Could you check a few things on this model? Use its own coordinates, in mm. Face numbers are marked on the shaded views. A direction names the side the tool comes from. Round coordinates to 2 decimals unless told otherwise and drop trailing zeros. Loops run counter-clockwise (first coordinate to the right, second up) from the corner with the lowest first, then second, coordinate; pieces in that order, holes last. Notation, with made-up numbers: (5.25, 46.5) -> (44.25, 46.5) arc R18 ccw to (44.25, 63.5) -> close; hole circle Ø9 at (70, 47.25). An arc over 180 degrees is marked (long way). One line per item, written item: value.
```python
from build123d import *

# Parameters (mm, degrees)
SKETCH1_W           = 69.85
SKETCH1_H           = 69.85
BOSS_EXTRUDE1_DEPTH = 381
SKETCH1_3_W         = 57.15
SKETCH1_3_H         = 57.15
CUT_EXTRUDE1_DEPTH  = 374.65
SKETCH2_R           = 6.35
CUT_EXTRUDE2_DEPTH  = 6.35


with BuildPart() as part:
    # Sketch1 → Boss-Extrude1 (new body)
    with BuildSketch(Plane.XY):
        with Locations((28.575, 28.575)):
            Rectangle(SKETCH1_W, SKETCH1_H)
    extrude(amount=BOSS_EXTRUDE1_DEPTH)

    # Sketch1<3> → Cut-Extrude1 (cut)
    with BuildSketch(Plane.XY):
        with Locations((28.575, 28.575)):
            Rectangle(SKETCH1_3_W, SKETCH1_3_H)
    extrude(amount=CUT_EXTRUDE1_DEPTH, mode=Mode.SUBTRACT)

    # Sketch2 → Cut-Extrude2 (cut)
    with BuildSketch(Plane.XZ.offset(6.35)):
        with Locations(Location((28.575, 349.25, 0), (0, 0, 270))):
            Circle(SKETCH2_R)
    extrude(amount=-CUT_EXTRUDE2_DEPTH, mode=Mode.SUBTRACT)


solid = part.part
```
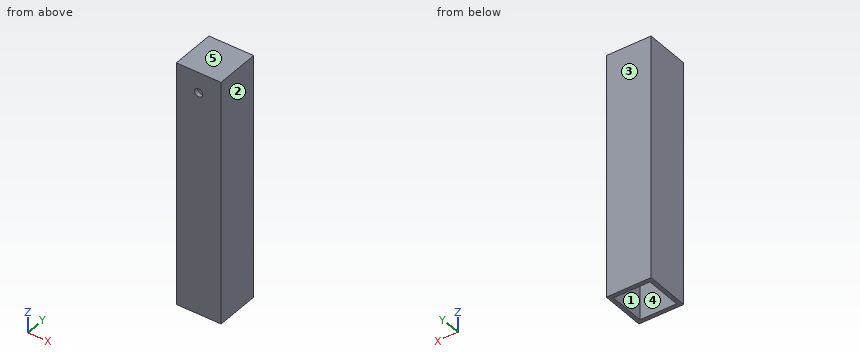
Item 1: If we mould it in two halves opening along X, with no side actions, what happens to the marked faces 1, 2 and 3? For each: released by +X, released by -X, zero draft, split by the parting line, or undercut.
Output:
face 1: undercut
face 2: released by +X
face 3: zero draft
Item 2: For the marked faces 4 and 5, which set-ups out of +Z, -Z, +X, -X, +Y, -Y let a thin tool reach every point of the face, with its end or its side?
Output:
face 4: -Z
face 5: +Z, +X, -X, +Y, -Y
Item 3: Will this pin go through, and if not, where does the flat tip stop? pin 1 Ø1 at (x, y) = (18.5, 31) entering from -Z.
Output:
pin 1: stops at z = 374.65
Item 4: If we section it at B-B on y = 19: List the corners of the cut face in (x, z) for me, plus the area to 3 significant figures.
Output:
outline: (-6.35, 0) -> (0, 0) -> (0, 374.65) -> (57.15, 374.65) -> (57.15, 0) -> (63.5, 0) -> (63.5, 381) -> (-6.35, 381) -> close
area: 5,200 mm²
Item 5: If we section it at D-D on z = 349.25: List the corners of the cut face in (x, y) for me (3 decimals).
Output:
outline: (-6.35, -6.35) -> (22.225, -6.35) -> (22.225, 0) -> (0, 0) -> (0, 57.15) -> (57.15, 57.15) -> (57.15, 0) -> (34.925, 0) -> (34.925, -6.35) -> (63.5, -6.35) -> (63.5, 63.5) -> (-6.35, 63.5) -> close
Item 6: I need wall thicknesses on line 1 (Y direction, x = 49.5, z = 288.5); line 2 (X direction, y = -3, z = 349). Which ranges of each line are inside material? Lowest first, please. Write a range as from..to.
Output:
line 1: y = -6.35..0, 57.15..63.5
line 2: x = -6.35..22.23, 34.92..63.5
Item 7: If we section it at A-A on z = 238: List the corners of the cut face in (x, y) for me.
Output:
outline: (-6.35, -6.35) -> (63.5, -6.35) -> (63.5, 63.5) -> (-6.35, 63.5) -> close; hole (0, 0) -> (57.15, 0) -> (57.15, 57.15) -> (0, 57.15) -> close
